```python
from build123d import *

# Parameters (mm, degrees)
ESQUISSE1_R             = 6
BOSS_EXTRU_1_DEPTH      = 15
ESQUISSE2_R             = 0.3
ENL_V_MAT_EXTRU_1_DEPTH = 3
ESQUISSE3_W             = 12.003336486
ESQUISSE3_H             = 20
BOSS_EXTRU_2_DEPTH      = 1


with BuildPart() as part:
    # Esquisse1 → Boss.-Extru.1 (new body)
    with BuildSketch(Plane.XY):
        Circle(ESQUISSE1_R)
    extrude(amount=BOSS_EXTRU_1_DEPTH)

    # Esquisse2 → Enlèv. mat.-Extru.1 (cut)
    with BuildSketch(Plane.XY.offset(15)):
        Circle(ESQUISSE2_R)
    extrude(amount=-ENL_V_MAT_EXTRU_1_DEPTH, mode=Mode.SUBTRACT)

    # Esquisse3 → Boss.-Extru.2 (add)
    with BuildSketch(Plane(origin=(0, 0, 0), x_dir=(1, 0, 0), z_dir=(0, 1, 0))):
        with Locations((0.001668243, 10)):
            Rectangle(ESQUISSE3_W, ESQUISSE3_H)
    extrude(amount=BOSS_EXTRU_2_DEPTH)


solid = part.part
```
The listing builds one solid part. Answer for the finished solid, in the listing's coordinates (mm). A direction names the side the tool comes from. Give positions to 0.01 mm unless a question says otherwise; leave off trailing zeros. Write each loop counter-clockwise with the first axis right and the second up, starting at its lowest first coordinate (ties: lowest second). Pieces come first, ordered by that corner, then holes. Notation, with made-up numbers: (4.5, -24) -> (56.5, -24) arc R24 cw to (56.5, -3) -> close; hole circle Ø8 at (89, 71). An arc over 180 degrees is marked (long way). Write item = value, one per line. Start each with the question number.
1) The part is cut by section C-C, the plane z = -5. Determine the outline of the cut face in (x, y), and give its area (3 significant figures).
2) Which of the six approach directions +Z, -Z, +X, -X, +Y, -Y give full straight-line access (tool end or side, diameter ignored) to faces 1 (the face through (0, 1, -10)), 2 (the face through (-6, 0.5, -9.9)), 3 (the face through (0, -2, 0))?
3) The part is cut by section D-D, the plane y = -4.75. Determine the outline of the cut face in (x, z).
4) The part is cut by section B-B, the plane x = 5. Determine the outline of the cut face in (y, z), and give its area (3 significant figures).
5) The part is cut by section A-A, the plane z = 13.5. Determine the outline of the cut face in (x, y), and give its area (3 significant figures).
6) Each of these flat-tipped pins is pushed along its axis until it touches: pin 1 (6 mm diameter, centred on x = 1.5, z = -11, fed in from +Y); pin 2 (1.5 mm diameter, centred on x = -3, y = -1, fed in from -Z); pin 3 (4 mm diameter, centred on y = -1, z = -12.5, fed in from +X); pin 4 (2 mm diameter, centred on x = -2, z = -10, fed in from -Y). Where does it stop, or does it pass through?
7) Straight lines are drawn through the part: line 1 along Y through (x, z) = (0, 13.2); line 2 along Z through (x, y) = (0, 1.5); line 3 along Y through (x, z) = (1, 2). For each, find the intervals that lie inside material, in ascending order.
Solutions:
q1.outline = (-6, 0) -> (6, 0) -> (6, 1) -> (-6, 1) -> close
q1.area = 12.0 mm²
q2.face_1 = -Z, +X, -X, +Y
q2.face_2 = +Z, -Z, -X, +Y, -Y
q2.face_3 = -Z, +X, -X, -Y
q3.outline = (-3.67, 0) -> (3.67, 0) -> (3.67, 15) -> (-3.67, 15) -> close
q4.outline = (-3.32, 0) -> (0, 0) -> (0, -20) -> (1, -20) -> (1, 0) -> (3.32, 0) -> (3.32, 15) -> (-3.32, 15) -> close
q4.area = 119 mm²
q5.outline = circle Ø12 at (0, 0); hole circle Ø0.6 at (0, 0)
q5.area = 113 mm²
q6.pin_1 = 1
q6.pin_2 = 0
q6.pin_3 = 6
q6.pin_4 = 0
q7.line_1 = -6 to -0.3, 0.3 to 6
q7.line_2 = 0 to 15
q7.line_3 = -5.92 to 5.92
